Autodesk Inventor part; units mm, degrees
ref_plane "YZ Plane" through (0, 0, 0) normal (1, 0, 0) x (0, 1, 0)
ref_plane "XZ Plane" through (0, 0, 0) normal (0, 1, 0) x (-1, 0, 0)
ref_plane "XY Plane" through (0, 0, 0) normal (0, 0, 1) x (1, 0, 0)
sketch "Sketch1" plane through (0, 0, 0) normal (0, 1, 0) x (-1, 0, 0)
  line L0 (0, 0) -> (62.2, 0)
  line L1 (62.2, 0) -> (62.2, -54.8)
  line L2 (62.2, -54.8) -> (0, -54.8)
  line L3 (0, -54.8) -> (0, 0)
  dimension "d0" = 54.8
  dimension "d1" = 62.2
extrude "Extrusion1" add sketch "Sketch1" along normal blind 19
sketch "Sketch2" plane through (0, 19, 0) normal (0, 1, 0) x (1, 0, 0)
  line L0 (-62.2, 54.8) -> (-62.2, 0)
  line L1 (0, 54.8) -> (-62.2, 54.8)
  point P0 (0, 0)
  point P1 (-59.7, 52.3)
  dimension "d4" = 2.5
  dimension "d5" = 2.5
hole "Hole1" at (-59.7, 19, -52.3) direction (0, -1, 0) diameter 3 end through all
ref_plane "Work Plane1" through (-62.2, 0, -27.4) normal (0, 0, 1) x (1, 0, 0)
ref_plane "Work Plane2" through (-31.1, 0, 0) normal (1, 0, 0) x (0, 0, -1)
mirror "Mirror1" about plane through (-62.2, 0, -27.4) normal (0, 0, 1) of "Hole1"
mirror "Mirror2" about plane through (-31.1, 0, 0) normal (1, 0, 0) of "Hole1", "Mirror1"
sketch "Sketch3" plane through (0, 19, 0) normal (0, 1, 0) x (1, 0, 0)
  line L0 (-47.9, 1) -> (-51.9, 1)
  line L1 (-51.9, 1) -> (-51.9, 17.4)
  line L2 (-51.9, 17.4) -> (-47.9, 17.4)
  line L3 (-47.9, 17.4) -> (-47.9, 1)
  line L4 (-62.2, 0) -> (0, 0)
  line L5 (-62.2, 54.8) -> (-62.2, 0)
  dimension "d13" = 4
  dimension "d14" = 16.4
  dimension "d15" = 1
  dimension "d16" = 10.3
extrude "Extrusion2" add sketch "Sketch3" along normal blind 28.6
sketch "Sketch4" plane through (0, 19, 0) normal (0, 1, 0) x (1, 0, 0)
  circle A0 centre (-5.7, 9) radius 2.75
  line L0 (-62.2, 0) -> (0, 0)
  line L1 (0, 0) -> (0, 54.8)
  dimension "d19" = 5.5
  dimension "d20" = 9
  dimension "d21" = 5.7
extrude "Extrusion3" cut sketch "Sketch4" against normal blind 10
properties part number "board"
Geometry: final body of the model. Coordinates: model frame, mm. A direction names the side the tool comes from. Round coordinates to 2 decimals unless told otherwise and drop trailing zeros. Order: outer loops, then holes, each group sorted by start corner. A loop starts at its lowest first (then second) coordinate and runs counter-clockwise, first axis right, second up. Notation, with made-up numbers: M -28,66 L 6,66 A13 cw 6,84 Z; hole C 61.25,-22.5 d1. An arc over 180 degrees is marked long. One line per item, written item: value.
(1) Reachability of faces 5 (the cylindrical face through (-3.08, 14.07, -9.83)), 6 (the flat face through (-50, 33, -1)), 7 (the flat face through (-50, 33, -17.4)) from +Z, -Z, +X, -X, +Y, -Y: full face, straight path, thin tool, end or side. Return the list, or none.
Result sheet:
face 5: +Y
face 6: +Z, +X, -X, +Y
face 7: -Z, +X, -X, +Y
(2) Pull-direction query (X, two-part tool) for faces 1 (the flat face through (-47.9, 33, -9)), 2 (the cylindrical face through (-1.6, 9.4, -53.5)), 3 (the flat face through (-6, 9, -9)), 4 (the flat face through (-51.9, 33, -9)); classes: pulls with the +X half, pulls with the -X half, needs draft (parallel to the pull), parting line crosses it, or undercut.
Result sheet:
face 1: pulls with the +X half
face 2: undercut
face 3: undercut
face 4: pulls with the -X half
(3) Cut plane C-C (z = -15.5). Return the cut outline in (x, y).
Result sheet:
outline: M -62.2,0 L 0,0 L 0,19 L -47.9,19 L -47.9,47.6 L -51.9,47.6 L -51.9,19 L -62.2,19 Z
(4) Cut plane B-B (y = 11). Return the cut outline in (x, z).
Result sheet:
outline: M -62.2,-54.8 L 0,-54.8 L 0,0 L -62.2,0 Z; hole C -59.7,-52.3 d3; hole C -59.7,-2.5 d3; hole C -5.7,-9 d5.5; hole C -2.5,-52.3 d3; hole C -2.5,-2.5 d3
(5) Line query: probe 1 along Z at (x, y) = (-59.7, 4.5); probe 2 along X at (y, z) = (11.5, -2.5); probe 3 along Z at (x, y) = (-5.7, 14.5). Output: solid intervals per line, ascending. Write a range as [from, to].
Result sheet:
probe 1: [-54.8, -53.8], [-50.8, -4], [-1, 0]
probe 2: [-62.2, -61.2], [-58.2, -4], [-1, 0]
probe 3: [-54.8, -11.75], [-6.25, 0]
(6) Pin query (flat end, axial travel): P1, Ø9, axis at x = -5.7, z = -9, coming from the +Y side; P2, Ø5, axis at y = 36.5, z = -10.5, coming from the +X side; P3, Ø4, axis at x = -2.5, z = -2.5, coming from the -Y side; P4, Ø2.5, axis at x = -2.5, z = -52.3, coming from the +Y side. Return the tip coordinate at first contact, or that it passes through.
Result sheet:
P1: y = 19
P2: x = -47.9
P3: y = 0
P4: through
(7) Cut plane D-D (x = -49.5). Return the cut outline in (y, z).
Result sheet:
outline: M 0,-54.8 L 19,-54.8 L 19,-17.4 L 47.6,-17.4 L 47.6,-1 L 19,-1 L 19,0 L 0,0 Z
(8) Cut plane A-A (z = -52.3). Return the cut outline in (x, y).
Result sheet:
outline: M -62.2,0 L -61.2,0 L -61.2,19 L -62.2,19 Z; M -58.2,0 L -4,0 L -4,19 L -58.2,19 Z; M -1,0 L 0,0 L 0,19 L -1,19 Z
